```python
from build123d import *

# Parameters (mm, degrees)
SKETCH1_R                   = 85
BOSS_EXTRUDE1_DEPTH         = 5
SKETCH14_R                  = 2
CUT_EXTRUDE2_DEPTH          = 133
SKETCH16_W                  = 35
SKETCH16_H                  = 4
CUT_EXTRUDE4_DEPTH          = 10
BOSS_EXTRUDE2_DEPTH         = 7
BOSS_EXTRUDE3_START         = 60
SKETCH20_R                  = 82
SKETCH20_R_2                = 78
BOSS_EXTRUDE3_DEPTH         = 60
BOSS_EXTRUDE4_START         = 60
BOSS_EXTRUDE4_DEPTH         = 60
SKETCH23_R                  = 1.5
CUT_EXTRUDE5_DEPTH          = 25
CUT_EXTRUDE6_DEPTH          = 110
CUT_EXTRUDE6_DEPTH_BACK     = 105
FILLET1_R                   = 3
SKETCH27_W                  = 14
SKETCH27_H                  = 14
BOSS_EXTRUDE5_DEPTH         = 5
CIRPATTERN1_COUNT           = 2
CIRPATTERN1_ANGLE           = 90
CIRPATTERN1_COPY_1_SKETCH_W = 14
CIRPATTERN1_COPY_1_SKETCH_H = 14
CIRPATTERN1_COPY_1_DEPTH    = 5
SKETCH29_R                  = 1.25
CUT_EXTRUDE7_DEPTH          = 5
CIRPATTERN2_COUNT           = 4


with BuildPart() as part:
    # Sketch1 → Boss-Extrude1 (new body)
    with BuildSketch(Plane(origin=(0, 0, 0), x_dir=(1, 0, 0), z_dir=(0, 1, 0))):
        with Locations(Location((0, 0, 0), (0, 0, 270))):
            Circle(SKETCH1_R)
    extrude(amount=BOSS_EXTRUDE1_DEPTH)

    # Sketch14 → Cut-Extrude2 (cut)
    with BuildSketch(Plane(origin=(0, 5, 0), x_dir=(1, 0, 0), z_dir=(0, 1, 0))):
        with Locations(Location((-53.033008589, 53.033008589, 0), (0, 0, 270))):
            Circle(SKETCH14_R)
        with Locations(Location((53.033008589, 53.033008589, 0), (0, 0, 270))):
            Circle(SKETCH14_R)
        with Locations(Location((53.033008589, -53.033008589, 0), (0, 0, 270))):
            Circle(SKETCH14_R)
        with Locations(Location((-53.033008589, -53.033008589, 0), (0, 0, 270))):
            Circle(SKETCH14_R)
    extrude(amount=-CUT_EXTRUDE2_DEPTH, mode=Mode.SUBTRACT)

    # Sketch16 → Cut-Extrude4 (cut)
    with BuildSketch(Plane(origin=(0, 5, 0), x_dir=(1, 0, 0), z_dir=(0, 1, 0))):
        Rectangle(SKETCH16_W, SKETCH16_H)
    extrude(amount=-CUT_EXTRUDE4_DEPTH, mode=Mode.SUBTRACT)

    # Sketch19 → Boss-Extrude2 (add)
    with BuildSketch(Plane(origin=(0, 5, 0), x_dir=(1, 0, 0), z_dir=(0, 1, 0))):
        with BuildLine():
            Line((75.342214451, 20.187885518), (80.171843582, 21.481980744))
            ThreePointArc((80.171843582, 21.481980744), (83, 0), (80.171843582, -21.481980744))
            Line((80.171843582, -21.481980744), (75.342214451, -20.187885518))
            ThreePointArc((75.342214451, -20.187885518), (78, 0), (75.342214451, 20.187885518))
        make_face()
        with BuildLine():
            Line((20.187885518, -75.342214451), (21.481980744, -80.171843582))
            ThreePointArc((21.481980744, -80.171843582), (0, -83), (-21.481980744, -80.171843582))
            Line((-21.481980744, -80.171843582), (-20.187885518, -75.342214451))
            ThreePointArc((-20.187885518, -75.342214451), (0, -78), (20.187885518, -75.342214451))
        make_face()
        with BuildLine():
            Line((-75.342214451, -20.187885518), (-80.171843582, -21.481980744))
            ThreePointArc((-80.171843582, -21.481980744), (-83, 0), (-80.171843582, 21.481980744))
            Line((-80.171843582, 21.481980744), (-75.342214451, 20.187885518))
            ThreePointArc((-75.342214451, 20.187885518), (-78, 0), (-75.342214451, -20.187885518))
        make_face()
        with BuildLine():
            Line((-20.187885518, 75.342214451), (-21.481980744, 80.171843582))
            ThreePointArc((-21.481980744, 80.171843582), (0, 83), (21.481980744, 80.171843582))
            Line((21.481980744, 80.171843582), (20.187885518, 75.342214451))
            ThreePointArc((20.187885518, 75.342214451), (0, 78), (-20.187885518, 75.342214451))
        make_face()
    extrude(amount=BOSS_EXTRUDE2_DEPTH)

    # Sketch20 → Boss-Extrude3 (add)
    with BuildSketch(Plane.XZ.offset(BOSS_EXTRUDE3_START)):
        with Locations(Location((0, 0, 0), (0, 0, 90))):
            Circle(SKETCH20_R)
        with Locations(Location((0, 0, 0), (0, 0, 270))):
            Circle(SKETCH20_R_2, mode=Mode.SUBTRACT)
    extrude(amount=-BOSS_EXTRUDE3_DEPTH)

    # Sketch22 → Boss-Extrude4 (add)
    with BuildSketch(Plane.XZ.offset(BOSS_EXTRUDE4_START)):
        with BuildLine():
            Line((-65, -7), (-65, -3))
            Line((-65, -3), (-77.942286341, -3))
            ThreePointArc((-77.942286341, -3), (-77.839472536, -5.00165126), (-77.685262438, -7))
            Line((-77.685262438, -7), (-65, -7))
        make_face()
        with BuildLine():
            ThreePointArc((-77.685262438, -7), (-77.839472536, -5.00165126), (-77.942286341, -3))
            Line((-77.942286341, -3), (-80.944425379, -3))
            ThreePointArc((-80.944425379, -3), (-80.845437043, -5.001530694), (-80.696964007, -7))
            Line((-80.696964007, -7), (-77.685262438, -7))
        make_face()
        with BuildLine():
            ThreePointArc((77.685262438, 7), (77.839472536, 5.00165126), (77.942286341, 3))
            Line((77.942286341, 3), (80.944425379, 3))
            ThreePointArc((80.944425379, 3), (80.845437043, 5.001530694), (80.696964007, 7))
            Line((80.696964007, 7), (77.685262438, 7))
        make_face()
        with BuildLine():
            Line((65, 3), (77.942286341, 3))
            ThreePointArc((77.942286341, 3), (77.839472536, 5.00165126), (77.685262438, 7))
            Line((77.685262438, 7), (65, 7))
            Line((65, 7), (65, 3))
        make_face()
        with BuildLine():
            Line((77.942286341, -3), (65, -3))
            Line((65, -3), (65, -7))
            Line((65, -7), (77.685262438, -7))
            ThreePointArc((77.685262438, -7), (77.839472536, -5.00165126), (77.942286341, -3))
        make_face()
        with BuildLine():
            Line((80.944425379, -3), (77.942286341, -3))
            ThreePointArc((77.942286341, -3), (77.839472536, -5.00165126), (77.685262438, -7))
            Line((77.685262438, -7), (80.696964007, -7))
            ThreePointArc((80.696964007, -7), (80.845437043, -5.001530694), (80.944425379, -3))
        make_face()
        with BuildLine():
            Line((-80.696964007, 7), (-65, 7))
            Line((-65, 7), (-65, 3))
            Line((-65, 3), (-80.944425379, 3))
            ThreePointArc((-80.944425379, 3), (-80.845437043, 5.001530694), (-80.696964007, 7))
        make_face()
    boss_extrude4 = extrude(amount=-BOSS_EXTRUDE4_DEPTH)

    # Sketch23 → Cut-Extrude5 (cut)
    with BuildSketch(Plane.XY.offset(7)):
        with Locations((-70, -30)):
            Circle(SKETCH23_R)
    cut_extrude5 = extrude(amount=-CUT_EXTRUDE5_DEPTH, mode=Mode.SUBTRACT)

    # Mirror1: Cut-Extrude5 across plane
    add(cut_extrude5.mirror(Plane(origin=(0, 0, 0), x_dir=(0, 0, 1), z_dir=(1, 0, 0))), mode=Mode.SUBTRACT)

    # Sketch25 → Cut-Extrude6 (cut, two sides: drawn at the far end of the back side and taken through both)
    with BuildSketch(Plane(origin=(0, 0, 0), x_dir=(0, 0, -1), z_dir=(1, 0, 0)).offset(-CUT_EXTRUDE6_DEPTH_BACK)):
        Polygon((-3, -27), (3, -27), (3, -33), (3, -43), (-3, -43), (-3, -33), align=None)
    extrude(amount=CUT_EXTRUDE6_DEPTH + CUT_EXTRUDE6_DEPTH_BACK, mode=Mode.SUBTRACT)

    # Fillet1
    fillet1_edges = [part.edges().sort_by_distance(p)[0] for p in [
        (-78, -27, 0),
        (78, -27, 0),
        (-78, -43, 0),
        (78, -43, 0),
    ]]
    fillet(fillet1_edges, radius=FILLET1_R)

    # Sketch27 → Boss-Extrude5 (add)
    with BuildSketch(Plane.XZ.offset(60)):
        with Locations((-72, 0)):
            Rectangle(SKETCH27_W, SKETCH27_H)
    boss_extrude5 = extrude(amount=-BOSS_EXTRUDE5_DEPTH)

    # Mirror2: Boss-Extrude5 across plane
    add(boss_extrude5.mirror(Plane(origin=(0, 0, 0), x_dir=(0, 0, 1), z_dir=(1, 0, 0))))

    # CirPattern1: Boss-Extrude4, Boss-Extrude5 ×2 about axis
    cirpattern1_axis = Axis((0, 0, 0), (0, -1, 0))
    add([boss_extrude4.rotate(cirpattern1_axis, i * CIRPATTERN1_ANGLE / (CIRPATTERN1_COUNT - 1)) for i in range(1, CIRPATTERN1_COUNT)])
    add([boss_extrude5.rotate(cirpattern1_axis, i * CIRPATTERN1_ANGLE / (CIRPATTERN1_COUNT - 1)) for i in range(1, CIRPATTERN1_COUNT)])

    # CirPattern1 copy 1 sketch → CirPattern1 copy 1 (add)
    with BuildSketch(Plane(origin=(0, -60, 0), x_dir=(0, 0, -1), z_dir=(0, -1, 0))):
        with Locations((-72, 0)):
            Rectangle(CIRPATTERN1_COPY_1_SKETCH_W, CIRPATTERN1_COPY_1_SKETCH_H)
    extrude(amount=-CIRPATTERN1_COPY_1_DEPTH)

    # Sketch29 → Cut-Extrude7 (cut)
    with BuildSketch(Plane.XZ.offset(60)):
        with Locations(Location((-72.5, 0, 0), (0, 0, 270))):
            Circle(SKETCH29_R)
    cut_extrude7 = extrude(amount=-CUT_EXTRUDE7_DEPTH, mode=Mode.SUBTRACT)

    # CirPattern2: Cut-Extrude7 ×4 about axis
    cirpattern2_axis = Axis((0, 0, 0), (0, 1, 0))
    for i in range(1, CIRPATTERN2_COUNT):
        add(cut_extrude7.rotate(cirpattern2_axis, i * 360 / CIRPATTERN2_COUNT), mode=Mode.SUBTRACT)


solid = part.part
```
The model under review builds one solid part; all positions refer to its coordinate system, in mm. A direction names the side the tool comes from. Round coordinates to 2 decimals unless told otherwise and drop trailing zeros. Order: outer loops, then holes, each group sorted by start corner. A loop starts at its lowest first (then second) coordinate and runs counter-clockwise, first axis right, second up. Notation, with made-up numbers: M 11.25,0.5 L 59.25,0.5 A24 ccw 59.25,39.5 Z; hole C 2,88.5 d10. An arc over 180 degrees is marked long. Use a Markdown table: item, result.
1) Insertion check: pin 1 (18.5 mm diameter, centred on x = -75, y = -39.5, fed in from -Z); pin 2 (1 mm diameter, centred on x = 38, y = -25.5, fed in from -Z); pin 3 (5 mm diameter, centred on x = 70, z = 0, fed in from +Y). Each pin has a flat end and moves straight along its axis. Give the tip position at first contact, or say it passes through.
Report:
| item | result |
|---|---|
| pin 1 | z = -49 |
| pin 2 | z = -72.92 |
| pin 3 | y = 5 |
2) Tool access review of faces 4 (the face through (0, -28, 78)), 5 (the face through (0, 3, -2)), 6 (the face through (0, 8, -83)): name each direction out of +Z, -Z, +X, -X, +Y, -Y from which nothing blocks a thin tool from reaching the whole face with its end or side.
Report:
| item | result |
|---|---|
| face 4 | none |
| face 5 | +Y, -Y |
| face 6 | -Z, +Y |
3) Wall thickness on line 1 along Y through (x, z) = (-70, -3.95); line 2 along Y through (x, z) = (66, -1.5); line 3 along X through (y, z) = (-57, -72): over which ranges is each line inside the solid? List them lowest first. Write a range as [from, to].
Report:
| item | result |
|---|---|
| line 1 | [-60, -31.5], [-28.5, 5] |
| line 2 | [-60, -55], [0, 5] |
| line 3 | [-39.24, -30], [-7, -1.15], [1.15, 7], [30, 39.24] |
4) Consider section C-C (x = -15). Write out the cut boundary in (y, z), then the cut area to 3 significant figures.
Report:
| item | result |
|---|---|
| outline | M -60,-80.62 L 0,-80.62 L 0,-83.67 L 5,-83.67 L 5,-81.63 L 12,-81.63 L 12,-76.54 L 5,-76.54 L 5,-2 L 0,-2 L 0,-76.54 L -60,-76.54 Z; M -60,76.54 L 0,76.54 L 0,2 L 5,2 L 5,76.54 L 12,76.54 L 12,81.63 L 5,81.63 L 5,83.67 L 0,83.67 L 0,80.62 L -60,80.62 Z |
| area | 1,380 mm^2 |
5) Consider section D-D (z = 29.5). Write out the cut boundary in (x, y), then the cut area to 3 significant figures.
Report:
| item | result |
|---|---|
| outline | M -79.72,0 L -76.51,0 L -76.51,-60 L -72.21,-60 L -72.21,0 L 72.21,0 L 72.21,-60 L 76.51,-60 L 76.51,0 L 79.72,0 L 79.72,5 L -79.72,5 Z |
| area | 1,310 mm^2 |
6) Draft analysis for pull direction X (two halves, no side actions). For faces 1 (the face through (0, 8, 78)), 2 (the face through (20.844, 8.451, -77.791)), 3 (the face through (0, 8, 83)), state which applies: released by +X, released by -X, zero draft, split by the parting line, or undercut.
Report:
| item | result |
|---|---|
| face 1 | undercut |
| face 2 | released by +X |
| face 3 | split by the parting line |
